The drawing under review shows one solid part. Ordinate dimensions are in mm from its lowest x, y, z. Round coordinates to 2 decimals unless told otherwise and drop trailing zeros. Order: outer loops, then holes, each group sorted by start corner. A loop starts at its lowest first (then second) coordinate and runs counter-clockwise, first axis right, second up. Notation, with made-up numbers: M 27,8.5 L 43,8.5 A19 cw 43,21.5 Z; hole C -28,78.5 d4. An arc over 180 degrees is marked long. Answer as a JSON object with one key per item and string values.
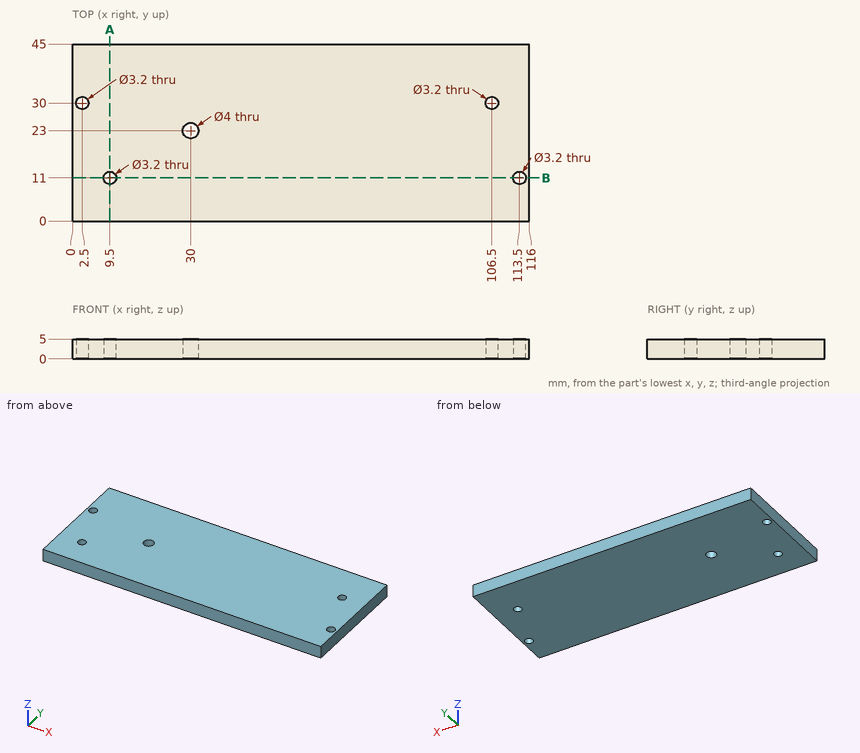
1) For L1, parallel to X at y = 30, z = 3.3; L2, parallel to X at y = 11, z = 2.1; L3, parallel to Y at x = 2.5, z = 3.8, list the stretches that pass through material, from the lowest coordinate up.
Geometry check:
{"L1": "x = 0 to 0.9, 4.1 to 104.9, 108.1 to 116", "L2": "x = 0 to 7.9, 11.1 to 111.9, 115.1 to 116", "L3": "y = 0 to 28.4, 31.6 to 45"}
2) Add section B-B on y = 11. State the section outline as (x, z) points, and give its area (3 significant figures).
Geometry check:
{"outline": "M 0,0 L 7.9,0 L 7.9,5 L 0,5 Z; M 11.1,0 L 111.9,0 L 111.9,5 L 11.1,5 Z; M 115.1,0 L 116,0 L 116,5 L 115.1,5 Z", "area": "548 mm²"}
3) Add section A-A on x = 9.5. State the section outline as (y, z) points, and give its area (3 significant figures).
Geometry check:
{"outline": "M 0,0 L 9.4,0 L 9.4,5 L 0,5 Z; M 12.6,0 L 45,0 L 45,5 L 12.6,5 Z", "area": "209 mm²"}
